from build123d import *

# Parameters (mm, degrees)
F1_DEPTH  = 190.5
F3_D      = 6.7564
F3_DEPTH  = 50.8
F3_TIP    = 2.0298273432
F5_D      = 6.7564
F7_D      = 6.7564
F9_D      = 6.7564
F11_D     = 6.7564
F11_DEPTH = 19.051
F13_D     = 6.7564


with BuildPart() as f1:
    # F0 (on Front) → F1 (new body)
    with BuildSketch(Plane.XZ):
        Polygon((114.3, -104.775), (95.25, -104.775), (19.05, -104.775), (-44.45, -104.775), (-95.25, -104.775), (-114.3, -104.775), (-114.3, -123.825), (114.3, -123.825), align=None)
        Polygon((95.25, -53.975), (95.25, -104.775), (114.3, -104.775), (114.3, 104.775), (95.25, 104.775), (95.25, 95.25), (95.25, 19.05), (95.25, 9.4333598495), (95.25, -28.575), align=None)
        Polygon((95.25, 104.775), (114.3, 104.775), (114.3, 123.825), (-114.3, 123.825), (-114.3, 104.775), (-95.25, 104.775), align=None)
        Polygon((-114.3, -104.775), (-95.25, -104.775), (-95.25, -53.975), (-95.25, -28.575), (-95.25, 22.225), (-95.25, 104.775), (-114.3, 104.775), align=None)
    extrude(amount=F1_DEPTH)

    # F3
    with Locations(Plane.XY.offset(123.825)):
        with Locations((-85.725, -38.1), (-85.725, -95.25), (-85.725, -152.4), (85.725, -152.4), (85.725, -95.25), (85.725, -38.1)):
            Hole(F3_D / 2, depth=F3_DEPTH)
            with Locations((0, 0, -(F3_DEPTH + F3_TIP / 2))):  # 118° drill point
                Cone(0, F3_D / 2, F3_TIP, mode=Mode.SUBTRACT)

    # F5 (through all)
    with Locations(Plane.XY.offset(123.825)):
        with Locations((-69.85, -13.4681584314), (69.85, -13.4681584314), (69.85, -177.8), (-69.85, -177.8)):
            Hole(F5_D / 2)

    # F7 (through all)
    with Locations(Plane.YZ.offset(114.3)):
        with Locations((-177.8, 41.275), (-12.7, 41.275), (-12.7, -79.375), (-177.8, -79.375)):
            Hole(F7_D / 2)

    # F9 (through all)
    with Locations(Plane.YZ.offset(114.3)):
        with Locations((-95.25, -44.45)):
            Hole(F9_D / 2)

    # F11 (through all, one way)
    with BuildSketch(Plane.XY.offset(-104.775)):
        with Locations((0, -95.25)):
            Circle(F11_D / 2)
    extrude(amount=-F11_DEPTH, mode=Mode.SUBTRACT)

    # F13 (through all)
    with Locations(Plane.YZ.offset(114.3)):
        with Locations((-146.05, -114.3), (-11.1125, 91.132421875), (-131.1710244843, -35.9210244843), (-167.0920489686, -71.8420489686)):
            Hole(F13_D / 2)


solid = f1.part
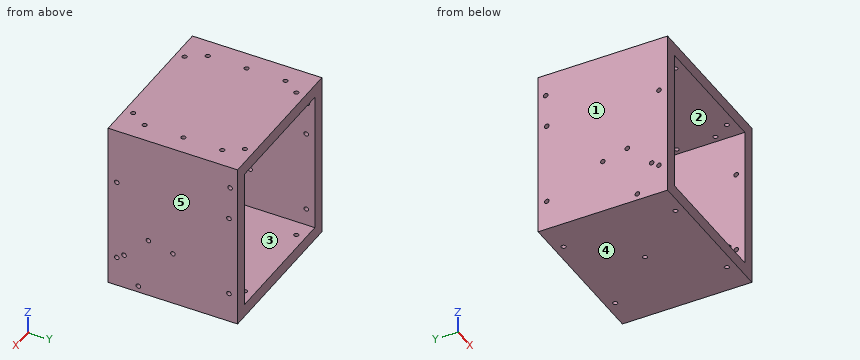
The model under review builds one solid part; all positions refer to its coordinate system, in mm. Face numbers are marked on the shaded views. A direction names the side the tool comes from. Round coordinates to 2 decimals unless told otherwise and drop trailing zeros. Order: outer loops, then holes, each group sorted by start corner. A loop starts at its lowest first (then second) coordinate and runs counter-clockwise, first axis right, second up. Notation, with made-up numbers: (84.25, 71.25) -> (88.25, 71.25) arc R18 ccw to (88.25, 103.25) -> close; hole circle Ø5 at (32, -38). An arc over 180 degrees is marked (long way). Write item = value, one per line. Start each with the question number.
Item 1: Consider section C-C on z = 8.5. Write out the cut boundary in (x, y).
Item 2: Consider section A-A on x = -69.85. Write out the cut boundary in (y, z) (3 decimals), plus the area to 3 significant figures.
Item 3: Consider section B-B on x = 0. Write out the cut boundary in (y, z) (3 decimals).
Item 4: For the marked faces 1 and 2, list the 3-axis set-ups (+Z, -Z, +X, -X, +Y, -Y) from which the entire face can be reached by the end or side of a thin tool; tool diameter is ignored.
Item 5: Mouldability with a two-part tool opening along Z and no side actions: class the marked faces 3, 4 and 5 as released by +Z, released by -Z, zero draft, split by the parting line, or undercut.
Item 6: Clearance check with a flat-ended pin moving along its axis: pin 1 Ø4 at (y, z) = (-167.09, -71.84) entering from +X. State where the tip first meets the part, or that it passes through.
Item 7: For line 1 along Z through (x, y) = (35.5, -11) (3 decimals); line 2 along X through (y, z) = (-140, -64); line 3 along Z through (x, y) = (104.25, -12.7) (3 decimals), list the stretches that pass through material, from the lowest coordinate up.
Item 8: Consider section D-D on x = 60.5. Write out the cut boundary in (y, z) (3 decimals).
Conclusion:
q1.outline = (-114.3, -190.5) -> (-95.25, -190.5) -> (-95.25, 0) -> (-114.3, 0) -> close; (95.25, -190.5) -> (114.3, -190.5) -> (114.3, 0) -> (95.25, 0) -> close
q2.outline = (-190.5, -123.825) -> (-181.178, -123.825) -> (-181.178, -104.775) -> (-190.5, -104.775) -> close; (-190.5, 104.775) -> (-181.178, 104.775) -> (-181.178, 123.825) -> (-190.5, 123.825) -> close; (-174.422, -123.825) -> (-16.846, -123.825) -> (-16.846, -104.775) -> (-174.422, -104.775) -> close; (-174.422, 104.775) -> (-16.846, 104.775) -> (-16.846, 123.825) -> (-174.422, 123.825) -> close; (-10.09, -123.825) -> (0, -123.825) -> (0, -104.775) -> (-10.09, -104.775) -> close; (-10.09, 104.775) -> (0, 104.775) -> (0, 123.825) -> (-10.09, 123.825) -> close; hole circle Ø6.756 at (-146.05, -114.3)
q2.area = 6,710 mm2
q3.outline = (-190.5, -123.825) -> (-98.628, -123.825) -> (-98.628, -104.775) -> (-190.5, -104.775) -> close; (-190.5, 104.775) -> (0, 104.775) -> (0, 123.825) -> (-190.5, 123.825) -> close; (-91.872, -123.825) -> (0, -123.825) -> (0, -104.775) -> (-91.872, -104.775) -> close; hole circle Ø6.756 at (-146.05, -114.3)
q4.face_1 = +Z, -Z, -X, +Y, -Y
q4.face_2 = +Y, -Y
q5.face_3 = undercut
q5.face_4 = released by -Z
q5.face_5 = zero draft
q6.pin_1 = through
q7.line_1 = -123.825 to -104.775, 104.775 to 123.825
q7.line_2 = -114.3 to -95.25, 95.25 to 114.3
q7.line_3 = -123.825 to -82.753, -75.997 to 37.897, 44.653 to 88.15, 94.114 to 123.825
q8.outline = (-190.5, -123.825) -> (0, -123.825) -> (0, -104.775) -> (-190.5, -104.775) -> close; (-190.5, 104.775) -> (0, 104.775) -> (0, 123.825) -> (-190.5, 123.825) -> close; hole circle Ø6.756 at (-146.05, -114.3)
